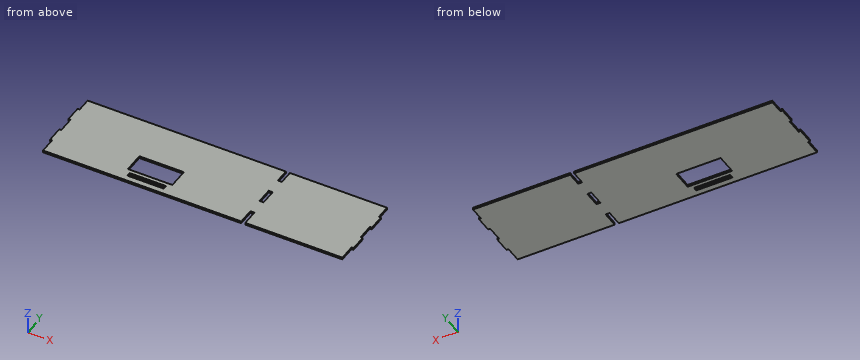
from build123d import *

# Parameters (mm, degrees)
ESQUISSE1_W             = 110
ESQUISSE1_H             = 50
BOSS_EXTRU_1_DEPTH      = 5
ENL_V_MAT_EXTRU_1_REACH = 776.952
ESQUISSE2_W             = 90
ESQUISSE2_H             = 10


with BuildPart() as part:
    # Esquisse1 → Boss.-Extru.1 (new body)
    # profile 1 of 2: a face of its own
    with BuildSketch(Plane.XY):
        Polygon((745, 120), (750, 120), (750, 160), (745, 160), (745, 195), (505, 195), (505, 160), (500, 160), (500, 120), (505, 120), (505, 80), (500, 80), (500, 40), (505, 40), (505, 0), (745, 0), (745, 40), (750, 40), (750, 80), (745, 80), align=None)
    # profile 2 of 2: a face of its own
    with BuildSketch(Plane.XY):
        Polygon((500, 120), (500, 160), (495, 160), (495, 195), (5, 195), (5, 160), (0, 160), (0, 120), (5, 120), (5, 80), (0, 80), (0, 40), (5, 40), (5, 0), (495, 0), (495, 40), (500, 40), (500, 80), (495, 80), (495, 120), align=None)
        with Locations((250, 60)):
            Rectangle(ESQUISSE1_W, ESQUISSE1_H, mode=Mode.SUBTRACT)
    extrude(amount=BOSS_EXTRU_1_DEPTH)

    # Esquisse2 → Enlèv. mat.-Extru.1 (cut, up to next)
    with BuildSketch(Plane.XY.offset(5), mode=Mode.PRIVATE) as enl_v_mat_extru_1_sk1:
        with Locations((250, 20)):
            Rectangle(ESQUISSE2_W, ESQUISSE2_H)
    enl_v_mat_extru_1_tool1 = extrude(enl_v_mat_extru_1_sk1.sketch, amount=-ENL_V_MAT_EXTRU_1_REACH, mode=Mode.PRIVATE) & part.part
    add(enl_v_mat_extru_1_tool1.solids().sort_by_distance((250, 20, 5))[0], mode=Mode.SUBTRACT)


solid = part.part
Read the model definition and answer for the solid it produces. Units are mm, in the model's axes. Coordinates: 2 decimals unless noted, no trailing zeros. Order: outer loops, then holes, each group sorted by start corner. A loop starts at its lowest first (then second) coordinate and runs counter-clockwise, first axis right, second up. Notation, with made-up numbers: M -5.75,-19 L 14.25,-19 A6 cw 14.25,-9 Z; hole C 7.25,1.25 d9. An arc over 180 degrees is marked long. Put each result on its own line as item: value. Start each with the question number.
Item 1: Section B-B, the plane y = 70.5 is taken. Determine the outline of the cut face in (x, z), plus the area to 3 significant figures.
Item 2: Section A-A, the plane x = 213 is taken. Determine the outline of the cut face in (y, z).
Item 3: Section C-C, the plane z = 1.45 is taken. Count the separate pieces of the cut face and the enclosed holes in it, plus the area to 3 significant figures.
Item 4: Consider probe 1 along X at (y, z) = (37, 2.2); probe 2 along X at (y, z) = (57, 2.25); probe 3 along X at (y, z) = (109.5, 0.9). Determine where each line is inside the solid, lowest interval first. Write a range as [from, to].
Item 5: Given pin 1 Ø3 at (x, y) = (486.5, 105) entering from -Z; pin 2 Ø2.5 at (y, z) = (170, 3.5) entering from +X; pin 3 Ø1.5 at (x, z) = (747.5, 1.5) entering from -Y; pin 4 Ø1.5 at (x, z) = (747.5, 3.5) entering from +Y, each flat-ended and moving along its own axis, determine where each tip first touches the part or whether it passes through.
Computed:
1. outline: M 0,0 L 195,0 L 195,5 L 0,5 Z; M 305,0 L 750,0 L 750,5 L 305,5 Z
1. area: 3,200 mm2
2. outline: M 0,0 L 15,0 L 15,5 L 0,5 Z; M 25,0 L 35,0 L 35,5 L 25,5 Z; M 85,0 L 195,0 L 195,5 L 85,5 Z
3. separate pieces: 1
3. enclosed holes: 3
3. area: 138,000 mm2
4. probe 1: x = [5, 195], [305, 495], [505, 745]
4. probe 2: x = [0, 195], [305, 750]
4. probe 3: x = [5, 495], [505, 745]
5. pin 1: stops at z = 0
5. pin 2: stops at x = 745
5. pin 3: stops at y = 40
5. pin 4: stops at y = 160
